from build123d import *

# Parameters (mm, degrees)
SKETCH_2_R               = 2.4
CUT_EXTRUDE_1_DEPTH      = 46.644495835
CHAMFER_1_SIZE           = 0.5
CHAMFER_2_SIZE           = 1
CUT_EXTRUDE_2_DEPTH      = 46.644495918
CUT_EXTRUDE_2_DEPTH_BACK = 46.644495918
SKETCH_3_R               = 1.4


with BuildPart() as part:
    # 스케치1 → 회전1 (revolve)
    with BuildSketch(Plane(origin=(0, 0, 0), x_dir=(0, 0, -1), z_dir=(1, 0, 0)), mode=Mode.PRIVATE) as revolve_1_sk:
        with BuildLine():
            Line((0, 13), (2, 13))
            Line((2, 13), (3.5, 12.75))
            Line((3.5, 12.75), (7.5, 12.75))
            ThreePointArc((7.5, 12.75), (8.019590324, 14.137023112), (8.996877215, 15.25))
            Line((8.996877215, 15.25), (37, 15.25))
            Line((37, 15.25), (37, 18.9))
            Line((37, 18.9), (0, 18.9))
            Line((0, 18.9), (0, 13))
        make_face()
    revolve(revolve_1_sk.sketch.rotate(Axis((0, 0, 0), (0, 0, -1)), 90), axis=Axis((0, 0, 0), (0, 0, -1)))

    # 스케치2 → 컷-돌출1 (cut, through all)
    with BuildSketch(Plane(origin=(0, 0, 0), x_dir=(1, 0, 0), z_dir=(0, 1, 0))):
        with Locations(Location((0, 25, 0), (0, 0, 270))):
            Circle(SKETCH_2_R)
    extrude(amount=-CUT_EXTRUDE_1_DEPTH, mode=Mode.SUBTRACT)

    # 모따기1
    chamfer_1_edges = [part.edges().sort_by_distance(p)[0] for p in [
        (-18.9, 0, -37),
    ]]
    chamfer(chamfer_1_edges, length=CHAMFER_1_SIZE)

    # 모따기2
    chamfer_2_edges = [part.edges().sort_by_distance(p)[0] for p in [
        (-18.9, 0, 0),
        (-15.25, 0, -37),
        (-13, 0, 0),
    ]]
    chamfer(chamfer_2_edges, length=CHAMFER_2_SIZE)

    # 스케치3 → 컷-돌출2 (cut, two sides: drawn at the far end of the back side and taken through both)
    with BuildSketch(Plane(origin=(0, 0, 0), x_dir=(0, 0, -1), z_dir=(1, 0, 0)).offset(-CUT_EXTRUDE_2_DEPTH_BACK)):
        with Locations((11, 0)):
            Circle(SKETCH_3_R)
    extrude(amount=CUT_EXTRUDE_2_DEPTH + CUT_EXTRUDE_2_DEPTH_BACK, mode=Mode.SUBTRACT)


solid = part.part
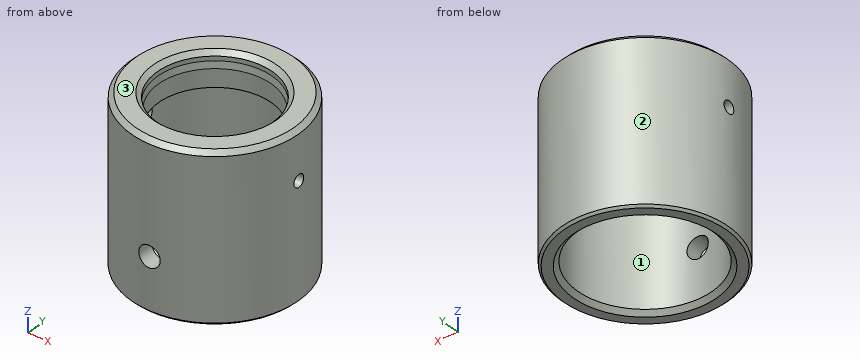
Input: part model. Units: mm. Frame: model coordinates. Face numbers are marked on the shaded views. Round coordinates to 2 decimals unless told otherwise and drop trailing zeros. Loops run counter-clockwise (first coordinate to the right, second up) from the corner with the lowest first, then second, coordinate; pieces in that order, holes last. Notation, with made-up numbers: M 72.5,88.25 L 95.5,88.25 A33 ccw 95.5,119.25 Z; hole C -10.5,19 d8. An arc over 180 degrees is marked long. Answer as CSV lines item,"result". Start each with the question number.
(1) Section A-A, the plane y = 0. State how many separate pieces and enclosed holes the cut face has, plus the area to 3 significant figures.
(2) First-contact query: pin 1 (12 mm diameter, centred on x = 14.5, z = -30, fed in from -Y); pin 2 (6 mm diameter, centred on x = 0, z = -25, fed in from +Y); pin 3 (4 mm diameter, centred on y = 9, z = -9.5, fed in from +X). Flat tips, straight axial feed; report the tip coordinate or a pass-through.
(3) Section B-B, the plane z = -11. Output: boundary loops of the cut face in (x, y), plus the area to 3 significant figures.
(4) Line query: line 1 (Y direction, x = 0, z = -28.5); line 2 (Y direction, x = 0, z = -1.45); line 3 (Y direction, x = 0, z = -27.25). Output: solid intervals per line, ascending. Write a range as [from, to].
(5) Draft query along Y for the marked faces 1, 2 and 3. Return one class per face: released by +Y, released by -Y, zero draft, split by the parting line, or undercut.
(6) Section C-C, the plane z = -22. Output: boundary loops of the cut face in (x, y), plus the area to 3 significant figures.
Values found:
1,separate pieces,"4"
1,enclosed holes,"0"
1,area,"285 mm²"
2,pin 1,"stops at y = -16.88"
2,pin 2,"stops at y = 18.9"
2,pin 3,"stops at x = 17.56"
3,outline,"M -18.85,-1.4 A18.9 ccw 18.85,-1.4 L 15.19,-1.4 A15.25 cw -15.19,-1.4 Z; M -18.85,1.4 L -15.19,1.4 A15.25 cw 15.19,1.4 L 18.85,1.4 A18.9 ccw Z"
3,area,"371 mm²"
4,line 1,"y = [-18.9, -15.25], [15.25, 18.9]"
4,line 2,"y = [-18.9, -13], [13, 18.9]"
4,line 3,"y = [15.25, 18.9]"
5,face 1,"undercut"
5,face 2,"split by the parting line"
5,face 3,"zero draft"
6,outline,"C 0,0 d37.8; hole C 0,0 d30.5"
6,area,"392 mm²"
